The model under review builds one solid part; all positions refer to its coordinate system, in mm. Face numbers are marked on the shaded views. A direction names the side the tool comes from. Coordinates: 2 decimals unless noted, no trailing zeros. Loops run counter-clockwise (first coordinate to the right, second up) from the corner with the lowest first, then second, coordinate; pieces in that order, holes last. Notation, with made-up numbers: M 66.5,34.25 L 121.5,34.25 A24 cw 121.5,62.25 Z; hole C 54.25,84.5 d5. An arc over 180 degrees is marked long. Use CSV: the item, a comma, the result in double quotes. Start each with the question number.
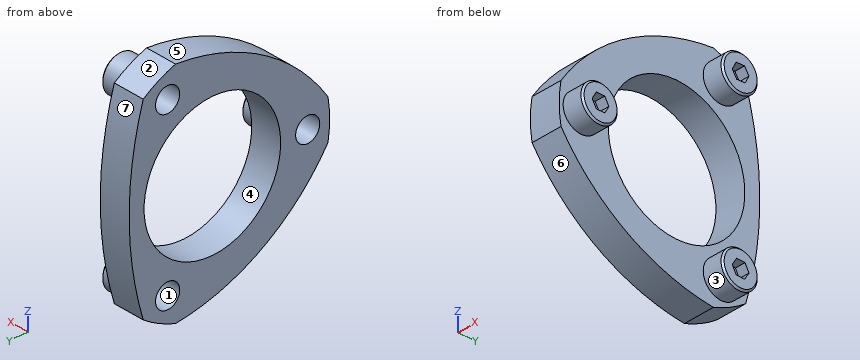
from build123d import *

# Parameters (mm, degrees)
SKETCH1_R           = 10.63625
BOSS_EXTRUDE1_DEPTH = 4.8387
HOLE1_D             = 3.7592
HOLE1_DEPTH         = 4.8387
HOLE2_D             = 3.7592
HOLE2_DEPTH         = 4.8387
HOLE3_D             = 3.7592
HOLE3_DEPTH         = 4.8387
CUT_EXTRUDE1_DEPTH  = 1.6129
CUT_EXTRUDE2_DEPTH  = 1.6129
CUT_EXTRUDE3_DEPTH  = 1.6129


with BuildPart() as part:
    # Sketch1 → Boss-Extrude1 (new body)
    with BuildSketch(Plane(origin=(0, 0, 0), x_dir=(0, 0, -1), z_dir=(1, 0, 0))):
        with BuildLine():
            ThreePointArc((-17.339461313, 5.732856195), (-12.932597366, -7.770688459), (-3.078572423, -18.001248584))
            ThreePointArc((-3.078572423, -18.001248584), (0, -18.2626), (3.078572423, -18.001248584))
            ThreePointArc((3.078572423, -18.001248584), (12.932597366, -7.770688459), (17.339461313, 5.732856195))
            ThreePointArc((17.339461313, 5.732856195), (16.242165379, 8.349528284), (14.752793477, 10.764647852))
            ThreePointArc((14.752793477, 10.764647852), (0, 12.954), (-14.752793477, 10.764647852))
            ThreePointArc((-14.752793477, 10.764647852), (-16.242165379, 8.349528284), (-17.339461313, 5.732856195))
        make_face()
        Circle(SKETCH1_R, mode=Mode.SUBTRACT)
    extrude(amount=BOSS_EXTRUDE1_DEPTH)

    # Hole1
    with Locations(Plane(origin=(4.8387, 0, 0), x_dir=(0, 0, -1), z_dir=(1, 0, 0))):
        with Locations((-13.108504848, 6.969915663)):
            Hole(HOLE1_D / 2, depth=HOLE1_DEPTH)

    # Sketch4 → Revolve1 (revolve)
    with BuildSketch(Plane(origin=(0, 0, 0), x_dir=(-1, 0, 0), z_dir=(0, -0.882947593, 0.469471563))):
        Polygon((-4.8387, -14.8463), (-4.8387, -17.6657), (-7.8105, -17.6657), (-8.0645, -17.4117), (-8.0645, -14.8463), align=None)
    revolve(axis=Axis((8.0645, 6.969915663, 13.108504848), (-1, 0, 0)))

    # Hole2
    with Locations(Plane(origin=(4.8387, 0, 0), x_dir=(0, 0, -1), z_dir=(1, 0, 0))):
        with Locations((13.108504848, 6.969915663)):
            Hole(HOLE2_D / 2, depth=HOLE2_DEPTH)

    # Sketch7 → Revolve2 (revolve)
    with BuildSketch(Plane(origin=(0, 0, 0), x_dir=(1, 0, 0), z_dir=(0, 0.882947593, 0.469471563))):
        Polygon((4.8387, 14.8463), (4.8387, 17.6657), (7.8105, 17.6657), (8.0645, 17.4117), (8.0645, 14.8463), align=None)
    revolve(axis=Axis((8.0645, 6.969915663, -13.108504848), (-1, 0, 0)))

    # Hole3
    with Locations(Plane(origin=(4.8387, 0, 0), x_dir=(0, 0, -1), z_dir=(1, 0, 0))):
        with Locations((0, -14.8463)):
            Hole(HOLE3_D / 2, depth=HOLE3_DEPTH)

    # Sketch10 → Revolve3 (revolve)
    with BuildSketch(Plane.XY):
        Polygon((4.8387, -14.8463), (4.8387, -12.0269), (7.8105, -12.0269), (8.0645, -12.2809), (8.0645, -14.8463), align=None)
    revolve(axis=Axis((8.0645, -14.8463, 0), (-1, 0, 0)))

    # Sketch11 → Cut-Extrude1 (cut)
    with BuildSketch(Plane(origin=(8.0645, 0, 0), x_dir=(0, 0, -1), z_dir=(1, 0, 0))):
        Polygon((-1.12776, -14.19518746), (-1.12776, -15.49741254), (0, -16.148525079), (1.12776, -15.49741254), (1.12776, -14.19518746), (0, -13.544074921), align=None)
    extrude(amount=-CUT_EXTRUDE1_DEPTH, mode=Mode.SUBTRACT)

    # Sketch12 → Cut-Extrude2 (cut)
    with BuildSketch(Plane(origin=(8.0645, 0, 0), x_dir=(0, 0, -1), z_dir=(1, 0, 0))):
        Polygon((11.958708349, 6.35855802), (13.063057848, 5.668483864), (14.212854347, 6.279841507), (14.258301347, 7.581273306), (13.153951848, 8.271347461), (12.004155349, 7.659989818), align=None)
    extrude(amount=-CUT_EXTRUDE2_DEPTH, mode=Mode.SUBTRACT)

    # Sketch13 → Cut-Extrude3 (cut)
    with BuildSketch(Plane(origin=(8.0645, 0, 0), x_dir=(0, 0, -1), z_dir=(1, 0, 0))):
        Polygon((-14.258301347, 7.581273306), (-14.212854347, 6.279841507), (-13.063057848, 5.668483864), (-11.958708349, 6.35855802), (-12.004155349, 7.659989818), (-13.153951848, 8.271347461), align=None)
    extrude(amount=-CUT_EXTRUDE3_DEPTH, mode=Mode.SUBTRACT)


solid = part.part
1. Add section B-B (y = 0). Write out the cut boundary in (x, z).
2. Insertion check: pin 1 Ø4 at (x, z) = (3.5, -7.5) entering from -Y; pin 2 Ø0.7 at (y, z) = (6.5, 13.5) entering from +X; pin 3 Ø1 at (x, y) = (7.5, -15) entering from +Z. Each pin has a flat end and moves straight along its axis. Give the tip position at first contact, or say it passes through.
3. To check wall thickness, follow line 1 along Y through (x, z) = (2.05, 0); line 2 along X through (y, z) = (-8, -9); line 3 along Z through (x, y) = (6.5, -14). State the ranges of each line that lie inside material, in increasing order.
4. Add section A-A (z = 9). Write out the cut boundary in (x, y).
5. For the marked faces 1, 2 and 3, list the 3-axis set-ups (+Z, -Z, +X, -X, +Y, -Y) from which the entire face can be reached by the end or side of a thin tool; tool diameter is ignored.
6. Add section D-D (x = 1.25). Write out the cut boundary in (y, z).
7. Add section C-C (x = 6). Write out the cut boundary in (y, z), plus the area to 3 significant figures.
8. Draft analysis for pull direction Z (two halves, no side actions). For the marked faces 4, 5, 6 and 7, state which applies: released by +Z, released by -Z, zero draft, split by the parting line, or undercut.
Solved:
1,outline,"M 0,-16.29 L 4.84,-16.29 L 4.84,-10.64 L 0,-10.64 Z; M 0,10.64 L 4.84,10.64 L 4.84,16.29 L 0,16.29 Z"
2,pin 1,"stops at y = -16.25"
2,pin 2,"stops at x = 6.45"
2,pin 3,"stops at z = 2.82"
3,line 1,"y = -18.26 to -16.73, -12.97 to -10.64, 10.64 to 12.95"
3,line 2,"x = 0 to 4.84"
3,line 3,"z = -2.69 to -0.79, 0.79 to 2.69"
4,outline,"M 0,-13.01 L 4.84,-13.01 L 4.84,-5.67 L 0,-5.67 Z; M 0,5.67 L 4.84,5.67 L 4.84,12.15 L 0,12.15 Z"
5,face 1,"-X"
5,face 2,"+Z, +X, -X, +Y"
5,face 3,"+X"
6,outline,"M -18,-3.08 A31.75 ccw 5.73,-17.34 A18.26 ccw 10.76,-14.75 A50.8 ccw 10.76,14.75 A18.26 ccw 5.73,17.34 A31.75 ccw -18,3.08 A18.26 ccw Z; hole C -14.85,0 d3.76; hole C 0,0 d21.27; hole C 6.97,-13.11 d3.76; hole C 6.97,13.11 d3.76"
7,outline,"C -14.85,0 d5.64; C 6.97,-13.11 d5.64; C 6.97,13.11 d5.64"
7,area,"74.9 mm^2"
8,face 4,"undercut"
8,face 5,"released by +Z"
8,face 6,"released by -Z"
8,face 7,"split by the parting line"
